Geometry: see drawing. Coordinates: mm, zero at the bounding-box minimum. Round coordinates to 2 decimals unless told otherwise and drop trailing zeros. Write each loop counter-clockwise with the first axis right and the second up, starting at its lowest first coordinate (ties: lowest second). Pieces come first, ordered by that corner, then holes. Notation, with made-up numbers: (16, 71) -> (75, 71) arc R25 ccw to (75, 90) -> close; hole circle Ø5 at (47.25, -26). An arc over 180 degrees is marked (long way). Write item = value, one per line. Start each with the question number.
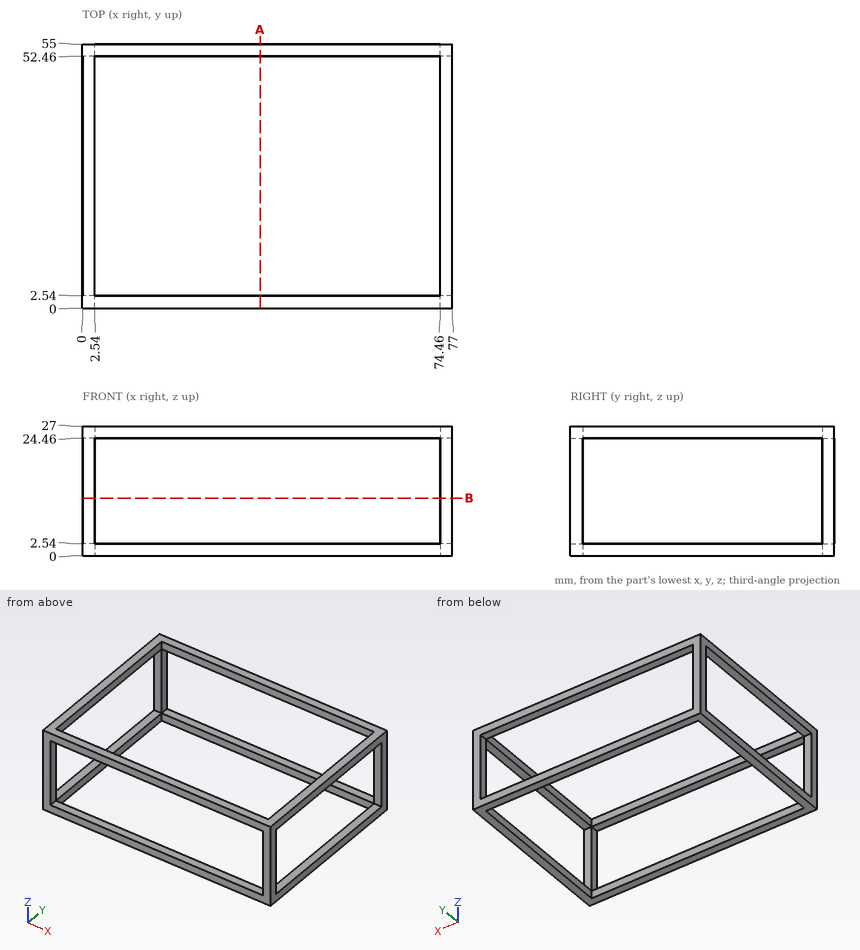
1. Section A-A (x = 37). Output: boundary loops of the cut face in (y, z).
2. Line query: line 1 along X through (y, z) = (32.5, 2.25); line 2 along Y through (x, z) = (7, 24.75). Output: solid intervals per line, ascending.
3. Section B-B (z = 12). Output: boundary loops of the cut face in (x, y), then the cut area to 3 significant figures.
Check sheet entries:
q1.outline = (0, 0) -> (2.54, 0) -> (2.54, 2.54) -> (0, 2.54) -> close; (0, 24.46) -> (2.54, 24.46) -> (2.54, 27) -> (0, 27) -> close; (52.46, 0) -> (55, 0) -> (55, 2.54) -> (52.46, 2.54) -> close; (52.46, 24.46) -> (55, 24.46) -> (55, 27) -> (52.46, 27) -> close
q2.line_1 = 0 to 2.54, 74.46 to 77
q2.line_2 = 0 to 2.54, 52.46 to 55
q3.outline = (0, 0) -> (2.54, 0) -> (2.54, 2.54) -> (0, 2.54) -> close; (0, 52.46) -> (2.54, 52.46) -> (2.54, 55) -> (0, 55) -> close; (74.46, 0) -> (77, 0) -> (77, 2.54) -> (74.46, 2.54) -> close; (74.46, 52.46) -> (77, 52.46) -> (77, 55) -> (74.46, 55) -> close
q3.area = 25.8 mm2
